Verification items for this drawing (mm, ordinates from the low corner). A direction names the side the tool comes from. Round coordinates to 2 decimals unless told otherwise and drop trailing zeros. Loops run counter-clockwise (first coordinate to the right, second up) from the corner with the lowest first, then second, coordinate; pieces in that order, holes last. Notation, with made-up numbers: M 6.5,28 L 62.5,28 A22 ccw 62.5,43 Z; hole C 27,73 d4. An arc over 180 degrees is marked long. Answer in a Markdown table with one row per item. Add a question column.
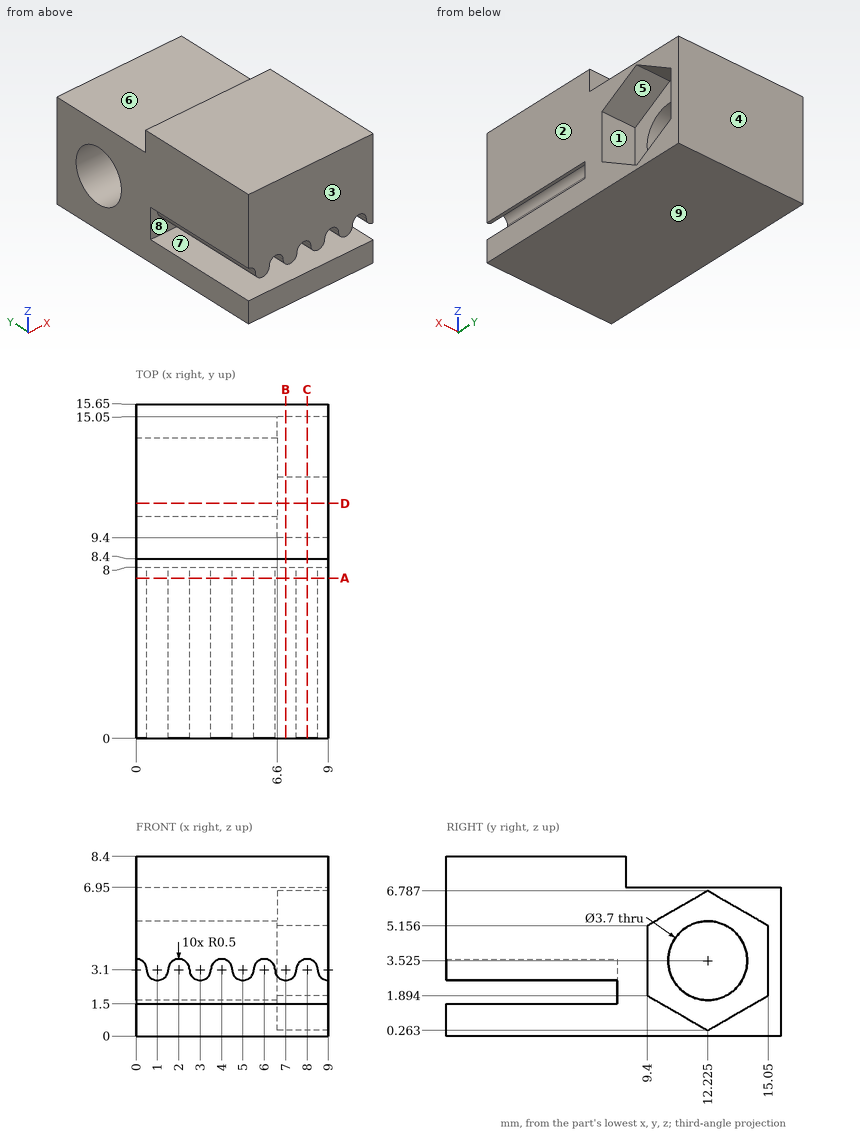
1) Draft check along Y on the marked faces 1, 2, 3 and 4. Enter one of: +Y half, -Y half, draft (parallel to the pull), parting line (faces both ways), or undercut.
2) Thickness scan on L1, parallel to Y at x = 4.75, z = 7.5; L2, parallel to Y at x = 7, z = 5.25; L3, parallel to X at y = 12.25, z = 1.25. Record the ranges inside material, lowest first. Write a range as [from, to].
3) Cross-section at C-C, the plane x = 8. Record the boundary of the cut face in (y, z) (3 decimals).
4) Set-up check for the marked faces 5, 6, 7, 8 and 9: record each of +Z, -Z, +X, -X, +Y, -Y from which the full face is reachable in a straight line by a thin tool's end or side.
5) Cross-section at A-A, the plane y = 7.5. Record the boundary of the cut face in (x, z), plus the area to 3 significant figures.
6) Cross-section at B-B, the plane x = 7. Record the boundary of the cut face in (y, z) (3 decimals), plus the area to 3 significant figures.
7) Go/stop test with a flat-tipped pin: pin 1 (2 mm diameter, centred on x = 5, y = 13.5, fed in from +Z). Record where the tip stops, or that it passes through.
8) Cross-section at D-D, the plane y = 11. Record the boundary of the cut face in (x, z).
Worked answers:
| question | item | result |
|---|---|---|
| 1 | face 1 | undercut |
| 1 | face 2 | draft |
| 1 | face 3 | -Y half |
| 1 | face 4 | +Y half |
| 2 | L1 | y = [0, 8.4] |
| 2 | L2 | y = [0, 9.56], [14.89, 15.65] |
| 2 | L3 | x = [0, 6.6] |
| 3 | outline | M 0,0 L 15.65,0 L 15.65,6.95 L 8.4,6.95 L 8.4,8.4 L 0,8.4 L 0,3.6 L 8,3.6 L 8,1.5 L 0,1.5 Z; hole M 9.4,1.894 L 12.225,0.263 L 15.05,1.894 L 15.05,5.156 L 12.225,6.787 L 9.4,5.156 Z |
| 4 | face 5 | +X |
| 4 | face 6 | +Z, +X, -X, +Y |
| 4 | face 7 | +X, -X, -Y |
| 4 | face 8 | -Y |
| 4 | face 9 | -Z, +X, -X, +Y, -Y |
| 5 | outline | M 0,0 L 9,0 L 9,1.5 L 0,1.5 Z; M 0,3.6 A0.5 cw 0.5,3.1 A0.5 ccw 1.5,3.1 A0.5 cw 2.5,3.1 A0.5 ccw 3.5,3.1 A0.5 cw 4.5,3.1 A0.5 ccw 5.5,3.1 A0.5 cw 6.5,3.1 A0.5 ccw 7.5,3.1 A0.5 cw 8.5,3.1 A0.5 ccw 9,2.6 L 9,8.4 L 0,8.4 Z |
| 5 | area | 61.2 mm2 |
| 6 | outline | M 0,0 L 15.65,0 L 15.65,6.95 L 8.4,6.95 L 8.4,8.4 L 0,8.4 L 0,2.6 L 8,2.6 L 8,1.5 L 0,1.5 Z; hole M 9.4,1.894 L 12.225,0.263 L 15.05,1.894 L 15.05,5.156 L 12.225,6.787 L 9.4,5.156 Z |
| 6 | area | 84.5 mm2 |
| 7 | pin 1 | stops at z = 6.95 |
| 8 | outline | M 0,0 L 9,0 L 9,0.97 L 6.6,0.97 L 6.6,2.14 L 0,2.14 Z; M 0,4.91 L 6.6,4.91 L 6.6,6.08 L 9,6.08 L 9,6.95 L 0,6.95 Z |
